Design review of the part built by this model. Coordinates are the model's own, in mm. A direction names the side the tool comes from. Coordinates: 2 decimals unless noted, no trailing zeros. Write each loop counter-clockwise with the first axis right and the second up, starting at its lowest first coordinate (ties: lowest second). Pieces come first, ordered by that corner, then holes. Notation, with made-up numbers: (-8, 64) - (3, 64) arc R25 ccw to (3, 88) - close; hole circle Ø4 at (22.5, 26). An arc over 180 degrees is marked (long way). Answer as CSV lines item,"result". Start each with the question number.
Q1. We need section D-D (x = 11.5). Write out the cut boundary in (y, z), plus the area to 3 significant figures.
Q2. We need section A-A (z = -8). Write out the cut boundary in (x, y), plus the area to 3 significant figures.
Q3. Machinability: for faces 4 (the face through (5, 1, 0)), 5 (the face through (-4.2, 1, -1)), 6 (the face through (-2, 1, -3)), which of the approach directions +Z, -Z, +X, -X, +Y, -Y give a long, thin tool a straight path to every point of the face, cutting with its end or side? Answer none if there is none.
Q4. For line 1 along X through (y, z) = (1.6, -8); line 2 along Z through (x, y) = (24.5, 1.15); line 3 along Z through (x, y) = (12, 0.8), list the stretches that pass through material, from the lowest coordinate up. Write a range as [from, to].
Q5. Mouldability with a two-part tool opening along Z and no side actions: class faces 1 (the face through (22.98, 1.01, -0.19)), 2 (the face through (5, 1, -16)), 3 (the face through (17, 0, -11)) as pulls with the +Z half, pulls with the -Z half, needs draft (parallel to the pull), parting line crosses it, or undercut.
Q6. Clearance check with flat-ended pins moving along their axes: pin 1 (12 mm diameter, centred on x = 16, z = -11.5, fed in from -Y); pin 2 (1 mm diameter, centred on x = -1.5, y = 0.5, fed in from +Z). State where each tip first meets the part, or that it passes through.
Q7. We need section B-B (y = 1.45). Write out the cut boundary in (x, z).
Q8. We need section C-C (x = 24.5). Write out the cut boundary in (y, z), plus the area to 3 significant figures.
Autodesk Inventor part; units mm, degrees
ref_plane "YZ Plane" through (0, 0, 0) normal (1, 0, 0) x (0, 1, 0)
ref_plane "XZ Plane" through (0, 0, 0) normal (0, 1, 0) x (-1, 0, 0)
ref_plane "XY Plane" through (0, 0, 0) normal (0, 0, 1) x (1, 0, 0)
sketch "Эскиз1" plane through (0, 0, 0) normal (0, 1, 0) x (-1, 0, 0)
  line L0 (0, 0) -> (4.2, 0)
  line L1 (4.2, 0) -> (4.2, -3)
  line L2 (4.2, -3) -> (0, -3)
  line L3 (0, -3) -> (0, -13)
  line L4 (4.2, -13) -> (0, -13)
  line L5 (4.2, -13) -> (4.2, -16)
  line L6 (4.2, -16) -> (0, -16)
  line L7 (0, -16) -> (-9.7125, -16)
  line L8 (-9.7125, -16) -> (-9.7125, 0)
  line L9 (-9.7125, 0) -> (4.2, 0)
  dimension "d0" = 4.2
  dimension "d1" = 10
  dimension "d2" = 3
  dimension "d3" = 3
extrude "Выдавливание1" add sketch "Эскиз1" along normal blind 2
sketch "Эскиз2" plane through (0, 2, 0) normal (0, 1, 0) x (1, 0, 0)
  line L0 (9.7125, 0) -> (9.7125, 16)
  line L1 (9.7125, 8) -> (24.7125, 8)
  circle A0 centre (24.7125, 8) radius 12.9007
  circle A1 centre (24.7125, 8) radius 8
  line L2 (9.7125, 16) -> (-4.2, 16)
  line L3 (9.7125, 16) -> (14.5918, 16)
  line L4 (-4.2, 0) -> (9.7125, 0)
  line L5 (9.7125, 0) -> (14.5918, 0)
  point P0 (0, 0)
  dimension "d6" = 15
extrude "Выдавливание2" add sketch "Эскиз2" against normal blind 2
fillet "Сопряжение1" radius 2 2 edges at (14.5918, 1, -16) (14.5918, 1, 0)
properties part number "kkekey"
Results list:
1,outline,"(0, -16) - (2, -16) - (2, 0) - (0, 0) - close"
1,area,"32.0 mm2"
2,outline,"(0, 0) - (16.71, 0) - (16.71, 2) - (0, 2) - close; (32.71, 0) - (37.61, 0) - (37.61, 2) - (32.71, 2) - close"
2,area,"43.2 mm2"
3,face 4,"+Z, -X, +Y, -Y"
3,face 5,"+Z, -Z, -X, +Y, -Y"
3,face 6,"-X, +Y, -Y"
4,line 1,"x = [0, 16.71], [32.71, 37.61]"
4,line 2,"z = [-20.9, -16], [0, 4.9]"
4,line 3,"z = [-16, 0]"
5,face 1,"undercut"
5,face 2,"pulls with the -Z half"
5,face 3,"needs draft"
6,pin 1,"stops at y = 0"
6,pin 2,"stops at z = 0"
7,outline,"(-4.2, -16) - (13.67, -16) arc R2 cw to (15.15, -16.66) arc R12.9 ccw (long way) to (15.15, 0.66) arc R2 cw to (13.67, 0) - (-4.2, 0) - (-4.2, -3) - (0, -3) - (0, -13) - (-4.2, -13) - close; hole circle Ø16 at (24.71, -8)"
8,outline,"(0, -20.9) - (2, -20.9) - (2, -16) - (0, -16) - close; (0, 0) - (2, 0) - (2, 4.9) - (0, 4.9) - close"
8,area,"19.6 mm2"
